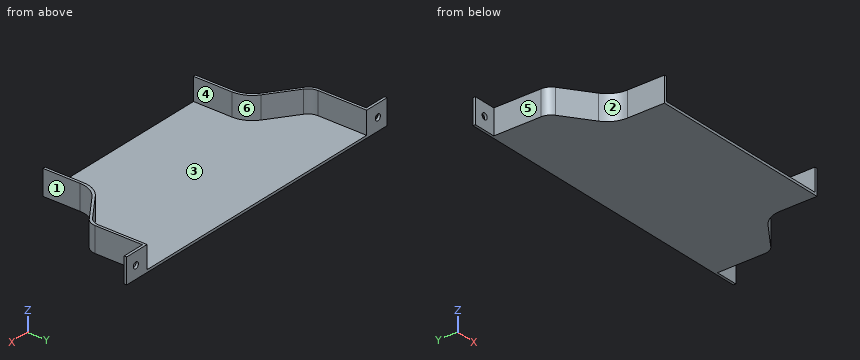
```python
from build123d import *

# Parameters (mm, degrees)
BOSS_EXTRU_1_DEPTH      = 20
ENL_V_MAT_EXTRU_2_DEPTH = 18
CONG_1_R                = 20
CONG_2_R                = 10
ESQUISSE7_W             = 20
ESQUISSE7_H             = 20
BOSS_EXTRU_2_DEPTH      = 2
ESQUISSE8_R             = 2.5
ENL_V_MAT_EXTRU_3_DEPTH = 10


with BuildPart() as part:
    # Esquisse1 → Boss.-Extru.1 (new body)
    with BuildSketch(Plane.XY):
        Polygon((110, 110), (-110, 110), (-110, 65), (-75, 40), (-75, 0), (75, 0), (75, 40), (110, 65), align=None)
    extrude(amount=BOSS_EXTRU_1_DEPTH)

    # Esquisse4 → Enlèv. mat.-Extru.2 (cut)
    with BuildSketch(Plane.XY.offset(20)):
        Polygon((-108, 181.485608489), (-108, 66.029235791), (-73, 41.029235791), (-73, -7.129747867), (73, -7.129747867), (73, 41.029235791), (108, 66.029235791), (108, 181.485608489), align=None)
    extrude(amount=-ENL_V_MAT_EXTRU_2_DEPTH, mode=Mode.SUBTRACT)

    # Congé1
    cong_1_edges = [part.edges().sort_by_distance(p)[0] for p in [
        (75, 40, 10),
        (-75, 40, 10),
        (73, 41.029235791, 11),
        (-73, 41.029235791, 11),
    ]]
    fillet(cong_1_edges, radius=CONG_1_R)

    # Congé2
    cong_2_edges = [part.edges().sort_by_distance(p)[0] for p in [
        (110, 65, 10),
        (-110, 65, 10),
        (-108, 66.029235791, 11),
        (108, 66.029235791, 11),
    ]]
    fillet(cong_2_edges, radius=CONG_2_R)

    # Esquisse7 → Boss.-Extru.2 (add)
    with BuildSketch(Plane(origin=(0, 110, 0), x_dir=(1, 0, 0), z_dir=(0, 1, 0))):
        with Locations((-118, -10)):
            Rectangle(ESQUISSE7_W, ESQUISSE7_H)
        with Locations((118, -10)):
            Rectangle(ESQUISSE7_W, ESQUISSE7_H)
    extrude(amount=-BOSS_EXTRU_2_DEPTH)

    # Esquisse8 → Enlèv. mat.-Extru.3 (cut)
    with BuildSketch(Plane.XZ.offset(-108)):
        with Locations(Location((119, 10, 0), (0, 0, 270))):
            Circle(ESQUISSE8_R)
        with Locations((-119, 10)):
            Circle(ESQUISSE8_R)
    extrude(amount=-ENL_V_MAT_EXTRU_3_DEPTH, mode=Mode.SUBTRACT)


solid = part.part
```
Work out the finished part from the listing and answer in its coordinate system (mm). Face numbers are marked on the shaded views. A direction names the side the tool comes from. Give positions to 0.01 mm unless a question says otherwise; leave off trailing zeros. Order: outer loops, then holes, each group sorted by start corner. A loop starts at its lowest first (then second) coordinate and runs counter-clockwise, first axis right, second up. Notation, with made-up numbers: M 54,80 L 73,80 A19 cw 73,109 Z; hole C 34.5,-13 d1. An arc over 180 degrees is marked long. Return JSON: item names as keys, results as strings.
1) Section C-C, the plane y = 80.5 is taken. Write down the section's boundary in (x, z).
Resolved:
{"outline": "M -110,0 L 110,0 L 110,20 L 108,20 L 108,2 L -108,2 L -108,20 L -110,20 Z"}
2) Straight lines are drawn through the part: line 1 along Z through (x, y) = (-119, 108.7); line 2 along X through (y, z) = (100, 7); line 3 along X through (y, z) = (30, 9.25). For each, find the intervals that lie inside material, in ascending order. Write a range as [from, to].
Resolved:
{"line 1": "[0, 7.5], [12.5, 20]", "line 2": "[-110, -108], [108, 110]", "line 3": "[-75, -73], [73, 75]"}
3) Section D-D, the plane x = -6 is taken. Write down the section's boundary in (y, z), plus the area to 3 significant figures.
Resolved:
{"outline": "M 0,0 L 110,0 L 110,2 L 0,2 Z", "area": "220 mm^2"}
4) Section A-A, the plane x = 119 is taken. Write down the section's boundary in (y, z), plus the area to 3 significant figures.
Resolved:
{"outline": "M 108,0 L 110,0 L 110,7.5 L 108,7.5 Z; M 108,12.5 L 110,12.5 L 110,20 L 108,20 Z", "area": "30.0 mm^2"}
5) Each of these flat-tipped pins is pushed along its axis until it touches: pin 1 (9 mm diameter, centred on x = 120, z = 14.5, fed in from -Y); pin 2 (8 mm diameter, centred on y = 33.5, z = 12, fed in from -X); pin 3 (10 mm diameter, centred on y = 97.5, z = 14, fed in from +X); pin 4 (1.5 mm diameter, centred on x = -19, y = 49, fed in from -Z). Where does it stop, or does it pass through?
Resolved:
{"pin 1": "y = 108", "pin 2": "x = -76.58", "pin 3": "x = 110", "pin 4": "z = 0"}
6) For a pull along X with two mould halves and no side action, classify the marked faces 1, 2 and 3 as +X half, -X half, draft (parallel to the pull), parting line (faces both ways), or undercut.
Resolved:
{"face 1": "+X half", "face 2": "-X half", "face 3": "undercut"}
7) A tool of negligible diameter and unlimited length cuts with its end or side. For the marked faces 4, 5 and 6, from which of +Z, -Z, +X, -X, +Y, -Y can it reach the whole face along a straight path? Write none if from no direction.
Resolved:
{"face 4": "+Z, +Y, -Y", "face 5": "+Z, -Z, -X, -Y", "face 6": "+Z, +Y"}
8) Section B-B, the plane z = 17.75 is taken. Write down the section's boundary in (x, y), plus the area to 3 significant figures.
Resolved:
{"outline": "M -128,108 L -110,108 L -110,70.15 A10 ccw -105.81,62.01 L -83.38,45.98 A20 cw -75,29.71 L -75,0 L -73,0 L -73,30.74 A20 ccw -81.38,47.01 L -103.81,63.04 A10 cw -108,71.18 L -108,110 L -128,110 Z; M 73,0 L 75,0 L 75,29.71 A20 cw 83.38,45.98 L 105.81,62.01 A10 ccw 110,70.15 L 110,108 L 128,108 L 128,110 L 108,110 L 108,71.18 A10 cw 103.81,63.04 L 81.38,47.01 A20 ccw 73,30.74 Z", "area": "584 mm^2"}
